from build123d import *

# Parameters (mm, degrees)
SKETCH_2_R   = 8
SKETCH_2_R_2 = 7


with BuildPart() as part:
    # По траектории1: sweep along a path in Эскиз1
    with BuildLine(Plane(origin=(0, 0, 0), x_dir=(1, 0, 0), z_dir=(0, 1, 0))) as sweep_1_path:
        Line((-275, -200), (-275, -80))
        ThreePointArc((-275, -80), (-251.568542495, -23.431457505), (-195, 0))
        Line((-195, 0), (0, 0))
    # Эскиз2 → По траектории1 (sweep)
    with BuildSketch(Plane(origin=(0, 0, 0), x_dir=(0, 0, -1), z_dir=(1, 0, 0))):
        Circle(SKETCH_2_R)
        Circle(SKETCH_2_R_2, mode=Mode.SUBTRACT)
    sweep(path=sweep_1_path.line)

    # Зеркальное отражение1: part across plane


with BuildPart() as part_1:
    add(part.part)
    add(part.part.mirror(Plane(origin=(0, 0, 0), x_dir=(0, 0, 1), z_dir=(1, 0, 0))))


solid = part_1.part
The listing builds one solid part. Answer for the finished solid, in the listing's coordinates (mm). A direction names the side the tool comes from. Round coordinates to 2 decimals unless told otherwise and drop trailing zeros. Order: outer loops, then holes, each group sorted by start corner. A loop starts at its lowest first (then second) coordinate and runs counter-clockwise, first axis right, second up. Notation, with made-up numbers: M -11,9.25 L 15,9.25 A16 cw 15,18.25 Z; hole C 2,56 d5. An arc over 180 degrees is marked long. Answer in a Markdown table with one row per item. Add a question column.
1) The part is cut by section B-B on z = 85. Determine the outline of the cut face in (x, y), plus the area to 3 significant figures.
2) The part is cut by section D-D on z = 58.5. Count the separate pieces of the cut face and the enclosed holes in it, plus the area to 3 significant figures.
3) The part is cut by section C-C on x = 169. Determine the outline of the cut face in (y, z), plus the area to 3 significant figures.
4) Flat-ended cylindrical pins translate along their axes: pin 1 Ø5 at (y, z) = (2.5, 20) entering from -X; pin 2 Ø1 at (y, z) = (3, 172) entering from +X; pin 3 Ø1 at (y, z) = (-4.5, 71.5) entering from -X; pin 4 Ø6 at (x, y) = (-103.5, 3) entering from -Z. Find the tip coordinate at first contact, or state that the pin passes through.
5) Which of the six approach directions +Z, -Z, +X, -X, +Y, -Y give full straight-line access (tool end or side, diameter ignored) to faces 4 (the face through (281.677, 2.103, 139.16)), 5 (the face through (279, -6, 200)), 6 (the face through (-2.73, -7.81, 1.73))?
6) Consider line 1 along Y through (x, z) = (-275, 170.5); line 2 along X through (y, z) = (-5.5, 87.5). Determine where each line is inside the solid, lowest interval first. Write a range as from..to.
7) Determine the mould class of faces 1 (the face through (2.73, -2.681, -6.466)), 2 (the face through (-282.63, 2.4, 139.16)), 3 (the face through (-279, -6, 200)) for opening direction X: pulls with the +X half, pulls with the -X half, needs draft (parallel to the pull), parting line crosses it, or undercut.
8) The part is cut by section A-A on y = 0. Determine the outline of the cut face in (x, z).
Findings below:
| question | item | result |
|---|---|---|
| 1 | outline | C -275,0 d16; C 275,0 d16; hole C -275,0 d14; hole C 275,0 d14 |
| 1 | area | 94.2 mm² |
| 2 | separate pieces | 2 |
| 2 | enclosed holes | 2 |
| 2 | area | 97.9 mm² |
| 3 | outline | C 0,0 d16; hole C 0,0 d14 |
| 3 | area | 47.1 mm² |
| 4 | pin 1 | stops at x = -261.26 |
| 4 | pin 2 | stops at x = 282.6 |
| 4 | pin 3 | stops at x = -281.52 |
| 4 | pin 4 | stops at z = -8 |
| 5 | face 4 | +Z |
| 5 | face 5 | +Z, +X, -X, +Y, -Y |
| 5 | face 6 | none |
| 6 | line 1 | y = -8..-7, 7..8 |
| 6 | line 2 | x = -280.81..-279.33, -270.67..-269.19, 269.19..270.67, 279.33..280.81 |
| 7 | face 1 | undercut |
| 7 | face 2 | undercut |
| 7 | face 3 | needs draft |
| 8 | outline | M -283,80 A88 ccw -195,-8 L 195,-8 A88 ccw 283,80 L 283,200 L 282,200 L 282,80 A87 cw 195,-7 L -195,-7 A87 cw -282,80 L -282,200 L -283,200 Z; M -268,80 A73 ccw -195,7 L 195,7 A73 ccw 268,80 L 268,200 L 267,200 L 267,80 A72 cw 195,8 L -195,8 A72 cw -267,80 L -267,200 L -268,200 Z |
